Input: part model. Units: mm. Frame: model coordinates. Face numbers are marked on the shaded views. Round coordinates to 2 decimals unless told otherwise and drop trailing zeros. Order: outer loops, then holes, each group sorted by start corner. A loop starts at its lowest first (then second) coordinate and runs counter-clockwise, first axis right, second up. Notation, with made-up numbers: (77.25, 43.25) - (116.25, 43.25) arc R26 cw to (116.25, 74.25) - close; hole circle Ø2 at (60.25, 34.25). An arc over 180 degrees is marked (long way). One line per item, written item: value. Start each with the question number.
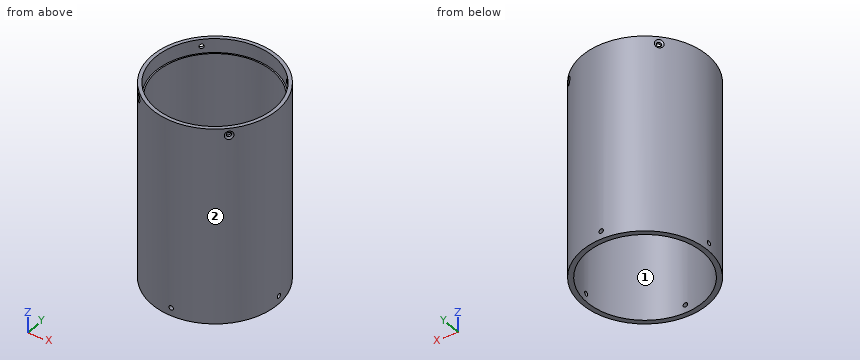
from build123d import *

# Parameters (mm, degrees)
ESQUISSE1_R                  = 44.5
BOSS_EXTRU_1_DEPTH           = 140
ESQUISSE2_R                  = 42
ENL_V_MAT_EXTRU_1_DEPTH      = 150
R_P_TITION_CIRCULAIRE1_COUNT = 4
ESQUISSE8_W                  = 1
ESQUISSE8_H                  = 130
R_P_TITION_CIRCULAIRE2_COUNT = 4


with BuildPart() as part:
    # Esquisse1 → Boss.-Extru.1 (new body)
    with BuildSketch(Plane.XY):
        Circle(ESQUISSE1_R)
    extrude(amount=BOSS_EXTRU_1_DEPTH)

    # Esquisse2 → Enlèv. mat.-Extru.1 (cut)
    with BuildSketch(Plane(origin=(0, 0, 0), x_dir=(-1, 0, 0), z_dir=(0, 0, -1))):
        Circle(ESQUISSE2_R)
    extrude(amount=-ENL_V_MAT_EXTRU_1_DEPTH, mode=Mode.SUBTRACT)

    # Esquisse5 → Dégagement M2.51 (revolve, cut)
    with BuildSketch(Plane(origin=(-31.466251763, 31.466251763, 135), x_dir=(-0.707106781, -0.707106781, 0), z_dir=(0, 0, 1))):
        Polygon((0, 0), (0, 15.931333959), (1.55, 15), (1.55, 0.83715789), (3, 0), align=None)
    d_gagement_m2_51 = revolve(axis=Axis((-35.956379823, 35.956379823, 135), (0.707106781, -0.707106781, 0)), mode=Mode.SUBTRACT)

    # Répétition circulaire1: Dégagement M2.51 ×4 about axis
    r_p_tition_circulaire1_axis = Axis((0, 0, 150), (0, 0, -1))
    for i in range(1, R_P_TITION_CIRCULAIRE1_COUNT):
        add(d_gagement_m2_51.rotate(r_p_tition_circulaire1_axis, i * 360 / R_P_TITION_CIRCULAIRE1_COUNT), mode=Mode.SUBTRACT)

    # Esquisse8 → Révolution1 (revolve)
    with BuildSketch(Plane(origin=(0, 0, 0), x_dir=(1, 0, 0), z_dir=(0, 1, 0))):
        with Locations((-41.5, -65)):
            Rectangle(ESQUISSE8_W, ESQUISSE8_H)
    revolve(axis=Axis((0, 0, -17.420915561), (0, 0, 1)))

    # Esquisse7 → Dégagement M2.52 (revolve, cut)
    with BuildSketch(Plane(origin=(-44.5, 0, 5.7), x_dir=(0, 0, 1), z_dir=(0, 1, 0))):
        Polygon((0, 0), (0, 20.931333959), (1.55, 20), (1.55, 0), align=None)
    d_gagement_m2_52 = revolve(axis=Axis((-50.85, 0, 5.7), (1, 0, 0)), mode=Mode.SUBTRACT)

    # Répétition circulaire2: Dégagement M2.52 ×4 about axis
    r_p_tition_circulaire2_axis = Axis((0, 0, 0), (0, 0, 1))
    for i in range(1, R_P_TITION_CIRCULAIRE2_COUNT):
        add(d_gagement_m2_52.rotate(r_p_tition_circulaire2_axis, i * 360 / R_P_TITION_CIRCULAIRE2_COUNT), mode=Mode.SUBTRACT)


solid = part.part
Item 1: Section query B-B on y = 25. Return loops of the section in (x, z), and give its area (3 significant figures).
Item 2: Pull-direction query (X, two-part tool) for the marked faces 1 and 2; classes: released by +X, released by -X, zero draft, split by the parting line, or undercut.
Item 3: First-contact query: pin 1 Ø1.5 at (y, z) = (18, 81.5) entering from -X; pin 2 Ø1.9 at (y, z) = (0, 5.7) entering from -X; pin 3 Ø1.5 at (x, z) = (-18.5, 56.5) entering from +Y; pin 4 Ø1.5 at (y, z) = (-14, 59) entering from -X. Flat tips, straight axial feed; report the tip coordinate or a pass-through.
Item 4: Section query C-C on z = 5.7. Return loops of the section in (x, y).
Item 5: Section query D-D on x = -39. Return loops of the section in (y, z).
Item 6: Line query: L1, parallel to Y at x = 0, z = 91.5; L2, parallel to Z at x = 0, y = -42.4. Output: solid intervals per line, ascending.
Item 7: Section query A-A on x = 0. Return loops of the section in (y, z), and give its area (3 significant figures).
Geometry results:
1. outline: (-36.81, 0) - (-32.5, 0) - (-32.5, 130) - (-33.75, 130) - (-33.75, 140) - (-36.81, 140) - close; (32.5, 0) - (36.81, 0) - (36.81, 140) - (33.75, 140) - (33.75, 130) - (32.5, 130) - close
1. area: 1,180 mm^2
2. face 1: undercut
2. face 2: split by the parting line
3. pin 1: stops at x = -41.02
3. pin 2: passes through
3. pin 3: stops at y = 40.81
3. pin 4: stops at x = -42.48
4. outline: (-44.47, -1.55) arc R44.5 ccw to (-1.55, -44.47) - (-1.55, -40.97) arc R41 cw to (-40.97, -1.55) - close; (-44.47, 1.55) - (-40.97, 1.55) arc R41 cw to (-1.55, 40.97) - (-1.55, 44.47) arc R44.5 ccw to start; (1.55, -44.47) arc R44.5 ccw to (44.47, -1.55) - (40.97, -1.55) arc R41 cw to (1.55, -40.97) - close; (1.55, 40.97) arc R41 cw to (40.97, 1.55) - (44.47, 1.55) arc R44.5 ccw to (1.55, 44.47) - close
5. outline: (-21.43, 0) - (-12.65, 0) - (-12.65, 130) - (-15.59, 130) - (-15.59, 140) - (-21.43, 140) - close; (12.65, 0) - (21.43, 0) - (21.43, 140) - (15.59, 140) - (15.59, 130) - (12.65, 130) - close
6. L1: y = -44.5 to -41, 41 to 44.5
6. L2: z = 0 to 4.15, 7.25 to 140
7. outline: (-44.5, 0) - (-41, 0) - (-41, 4.15) - (-44.5, 4.15) - close; (-44.5, 7.25) - (-41, 7.25) - (-41, 130) - (-42, 130) - (-42, 140) - (-44.5, 140) - close; (41, 0) - (44.5, 0) - (44.5, 4.15) - (41, 4.15) - close; (41, 7.25) - (44.5, 7.25) - (44.5, 140) - (42, 140) - (42, 130) - (41, 130) - close
7. area: 938 mm^2
